```python
from build123d import *

# Parameters (mm, degrees)
SKETCH1_R           = 3.1
BOSS_EXTRUDE1_DEPTH = 3
BOSS_EXTRUDE2_START = 3
SKETCH1_5_R         = 11
BOSS_EXTRUDE2_DEPTH = 15
CHAMFER1_SIZE       = 0.75


with BuildPart() as part:
    # Sketch1 → Boss-Extrude1 (new body)
    with BuildSketch(Plane(origin=(0, 0, 0), x_dir=(1, 0, 0), z_dir=(0, 1, 0))):
        Polygon((24, 12), (24, -12), (12, -12), (12, -24), (-12, -24), (-12, -12), (-24, -12), (-24, 12), (-12, 12), (-12, 24), (12, 24), (12, 12), align=None)
        with Locations(Location((17, 0, 0), (0, 0, 270))):
            Circle(SKETCH1_R, mode=Mode.SUBTRACT)
        with Locations(Location((0, -17, 0), (0, 0, 270))):
            Circle(SKETCH1_R, mode=Mode.SUBTRACT)
        with Locations(Location((0, 17, 0), (0, 0, 270))):
            Circle(SKETCH1_R, mode=Mode.SUBTRACT)
        with Locations(Location((-17, 0, 0), (0, 0, 270))):
            Circle(SKETCH1_R, mode=Mode.SUBTRACT)
    extrude(amount=BOSS_EXTRUDE1_DEPTH)

    # Sketch1<5> → Boss-Extrude2 (add)
    with BuildSketch(Plane(origin=(0, 0, 0), x_dir=(1, 0, 0), z_dir=(0, 1, 0)).offset(BOSS_EXTRUDE2_START)):
        with Locations(Location((0, 0, 0), (0, 0, 270))):
            Circle(SKETCH1_5_R)
    extrude(amount=BOSS_EXTRUDE2_DEPTH)

    # Sketch3 → Cut-Revolve3 (revolve, cut)
    with BuildSketch(Plane.XY, mode=Mode.PRIVATE) as cut_revolve3_sk:
        with BuildLine():
            Line((0, 18), (10.25, 18))
            ThreePointArc((10.25, 18), (7.247844507, 10.752155493), (0, 7.75))
            Line((0, 7.75), (0, 18))
        make_face()
    revolve(cut_revolve3_sk.sketch.rotate(Axis((0, 18, 0), (0, -1, 0)), 180), axis=Axis((0, 18, 0), (0, -1, 0)), mode=Mode.SUBTRACT)

    # Chamfer1
    chamfer1_edges = [part.edges().sort_by_distance(p)[0] for p in [
        (0, 18, -11),
    ]]
    chamfer(chamfer1_edges, length=CHAMFER1_SIZE - 0.0001)  # a hair under: the kernel refuses the full size


solid = part.part
```
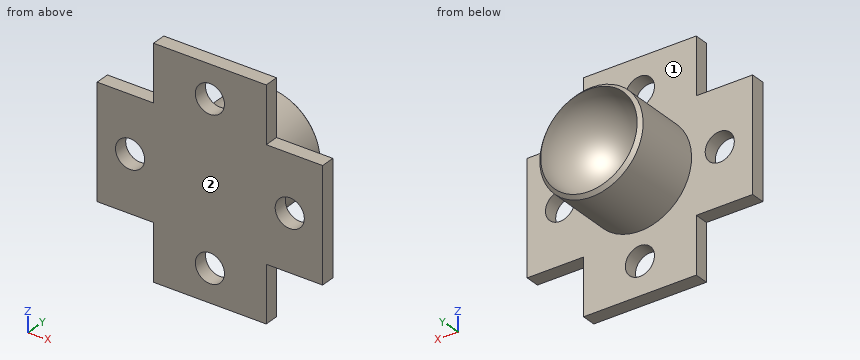
Design review of the part built by this model. Coordinates are the model's own, in mm. Face numbers are marked on the shaded views. A direction names the side the tool comes from. Round coordinates to 2 decimals unless told otherwise and drop trailing zeros. Write each loop counter-clockwise with the first axis right and the second up, starting at its lowest first coordinate (ties: lowest second). Pieces come first, ordered by that corner, then holes.
Item 1: For the marked faces 1 and 2, list the 3-axis set-ups (+Z, -Z, +X, -X, +Y, -Y) from which the entire face can be reached by the end or side of a thin tool; tool diameter is ignored.
Item 2: We need section C-C on x = 17. Write out the cut boundary in (y, z).
Item 3: For probe 1 along X at (y, z) = (1.7, 0); probe 2 along X at (y, z) = (1.75, 17); probe 3 along Z at (x, y) = (5, 13), list the stretches that pass through material, from the lowest coordinate up.
Item 4: We need section A-A on x = 0. State how many separate pieces and enclosed holes the cut face has, and give its area (3 significant figures).
Item 5: Clearance check with flat-ended pins moving along their axes: pin 1 Ø1.5 at (y, z) = (1, 18.5) entering from +X; pin 2 Ø2 at (y, z) = (13, 8.5) entering from +X; pin 3 Ø5 at (x, z) = (15, -13) entering from +Y. State where each tip first meets the part, or that it passes through.
Item 6: We need section B-B on z = 17. Write out the cut boundary in (x, y).
Returned:
1. face 1: +Y
1. face 2: +Z, -Z, +X, -X, -Y
2. outline: (0, -12) - (3, -12) - (3, -3.1) - (0, -3.1) - close; (0, 3.1) - (3, 3.1) - (3, 12) - (0, 12) - close
3. probe 1: x = -24 to -20.1, -13.9 to 13.9, 20.1 to 24
3. probe 2: x = -12 to -3.1, 3.1 to 12
3. probe 3: z = -9.8 to -7.42, 7.42 to 9.8
4. separate pieces: 3
4. enclosed holes: 0
4. area: 271 mm2
5. pin 1: stops at x = 12
5. pin 2: stops at x = 8.05
5. pin 3: stops at y = 3
6. outline: (-12, 0) - (-3.1, 0) - (-3.1, 3) - (-12, 3) - close; (3.1, 0) - (12, 0) - (12, 3) - (3.1, 3) - close
